The figure shows three views and two pictorial views of one solid part (mm, origin at its lowest corner). Answer the questions. A direction names the side the tool comes from. Coordinates: 2 decimals unless noted, no trailing zeros. Loops run counter-clockwise (first coordinate to the right, second up) from the corner with the lowest first, then second, coordinate; pieces in that order, holes last.
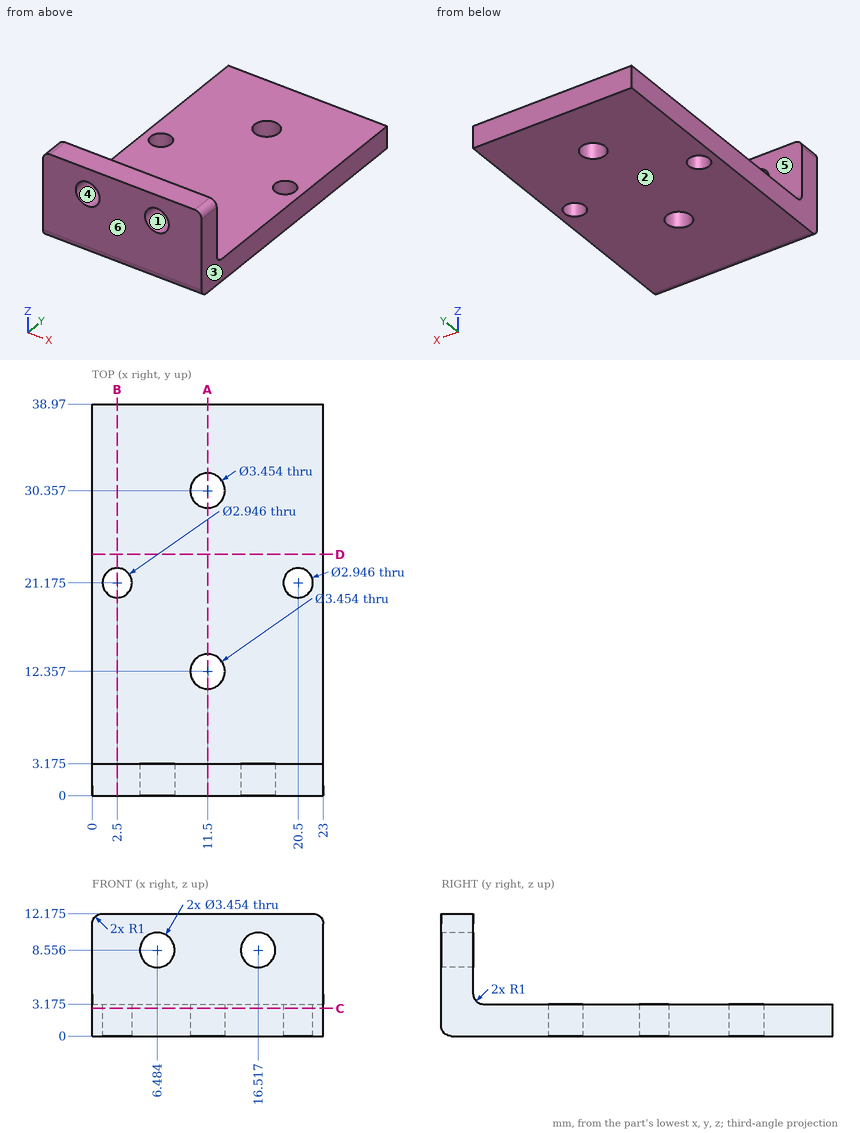
Q1. A cutting plane is placed at A-A (x = 11.5). Give the vertices of the cut face in (y, z) (1 decimal), then the cut area to 3 significant figures.
Findings below:
outline: (0, 1) arc R1 ccw to (1, 0) - (10.6, 0) - (10.6, 3.2) - (4.2, 3.2) arc R1 cw to (3.2, 4.2) - (3.2, 12.2) - (0, 12.2) - close; (14.1, 0) - (28.6, 0) - (28.6, 3.2) - (14.1, 3.2) - close; (32.1, 0) - (39, 0) - (39, 3.2) - (32.1, 3.2) - close
area: 130 mm2
Q2. Straight lines are drawn through the part: probe 1 along Y at (x, z) = (11.5, 1.7) (1 decimal); probe 2 along X at (y, z) = (2.5, 10) (1 decimal); probe 3 along Y at (x, z) = (2.5, 1.1). For each, find the intervals that lie inside material, in ascending order.
Findings below:
probe 1: y = 0 to 10.6, 14.1 to 28.6, 32.1 to 39
probe 2: x = 0 to 5.5, 7.4 to 15.6, 17.5 to 23
probe 3: y = 0 to 19.7, 22.65 to 38.97
Q3. A cutting plane is placed at B-B (x = 2.5). Give the vertices of the cut face in (y, z) (1 decimal), then the cut area to 3 significant figures.
Findings below:
outline: (0, 1) arc R1 ccw to (1, 0) - (19.7, 0) - (19.7, 3.2) - (4.2, 3.2) arc R1 cw to (3.2, 4.2) - (3.2, 12.2) - (0, 12.2) - close; (22.6, 0) - (39, 0) - (39, 3.2) - (22.6, 3.2) - close
area: 143 mm2
Q4. A cutting plane is placed at C-C (z = 2.75). Give the vertices of the cut face in (x, y) (1 decimal).
Findings below:
outline: (0, 0) - (23, 0) - (23, 39) - (0, 39) - close; hole circle Ø2.9 at (2.5, 21.2); hole circle Ø3.5 at (11.5, 12.4); hole circle Ø3.5 at (11.5, 30.4); hole circle Ø2.9 at (20.5, 21.2)
Q5. Which of the six approach directions +Z, -Z, +X, -X, +Y, -Y give full straight-line access (tool end or side, diameter ignored) to the marked faces 5 and 6?
Findings below:
face 5: +Z, +X, -X, +Y
face 6: +Z, -Z, +X, -X, -Y
Q6. Determine the mould class of the marked faces 1, 2, 3 and 4 for opening direction X: +X half, -X half, draft (parallel to the pull), parting line (faces both ways), or undercut.
Findings below:
face 1: undercut
face 2: draft
face 3: +X half
face 4: undercut
Q7. A cutting plane is placed at D-D (y = 24). Give the vertices of the cut face in (x, z) (1 decimal).
Findings below:
outline: (0, 0) - (23, 0) - (23, 3.2) - (0, 3.2) - close
Q8. Flat-ended cylindrical pins translate along their axes: pin 1 Ø2.5 at (x, y) = (20.5, 21.175) entering from +Z; pin 2 Ø3.5 at (x, y) = (2.5, 21.175) entering from +Z (1 decimal); pin 3 Ø4 at (x, z) = (18.5, 9) entering from +Y (1 decimal). Find the tip coordinate at first contact, or state that the pin passes through.
Findings below:
pin 1: passes through
pin 2: stops at z = 3.2
pin 3: stops at y = 3.2
